Check sheet for the modelled part. Datum: model origin and axes. Units: mm. A direction names the side the tool comes from. Coordinates: 2 decimals unless noted, no trailing zeros. Loops run counter-clockwise (first coordinate to the right, second up) from the corner with the lowest first, then second, coordinate; pieces in that order, holes last.
Autodesk Inventor part; units mm, degrees
ref_plane "YZ Plane" through (0, 0, 0) normal (1, 0, 0) x (0, 1, 0)
ref_plane "XZ Plane" through (0, 0, 0) normal (0, 1, 0) x (-1, 0, 0)
ref_plane "XY Plane" through (0, 0, 0) normal (0, 0, 1) x (1, 0, 0)
sketch "Sketch1" plane through (0, 0, 0) normal (0, 0, 1) x (1, 0, 0)
  circle A0 centre (0, 0) radius 4
  line L0 (-0.0635, 3.5) -> (1.9365, 3.5)
  line L1 (-0.0635, 3.5) -> (2, 3.5) construction
  line L2 (1.9365, 3.5) -> (-1.9365, 3.5)
  line L3 (0, -3.5) -> (1.9365, -3.5)
  line L4 (1.9365, -3.5) -> (-1.9365, -3.5)
  dimension "d0" = 8
  dimension "d1" = 2
  dimension "d2" = 0
extrude "Extrusion1" add sketch "Sketch1" along normal blind 3 contours A0 L3 L4 L2 L0
sketch "Sketch2" plane through (0, 0, 3) normal (0, 0, 1) x (1, 0, 0)
  circle A0 centre (0, 0) radius 2.5
  dimension "d5" = 5
extrude "Extrusion2" add sketch "Sketch2" along normal blind 53
sketch "Sketch3" plane through (0, 0, 56) normal (0, 0, 1) x (1, 0, 0)
  arc A0 (-1.9365, 3.5) -> (-1.9365, -3.5) centre (0, 0) ccw
  circle A1 centre (0, 0) radius 2
  dimension "d8" = 4
extrude "Extrusion3" cut sketch "Sketch3" against normal blind 8
properties part number "Rotation Pin"
(1) Section check C-C, the plane z = 38. Enter the section's corners in (x, y).
(2) Scan lines: line 1 along Y through (x, z) = (0, 52.5); line 2 along Z through (x, y) = (2.75, 2); line 3 along Y through (x, z) = (0, 5.5). Record each from-to range of solid material in increasing order.
(3) Set-up check for faces 4 (the face through (-0.54, 2.44, 29.13)), 5 (the face through (0, 0, 0)): record each of +Z, -Z, +X, -X, +Y, -Y from which the full face is reachable in a straight line by a thin tool's end or side.
(4) Gauge pin test, flat ends, axial feed: P1, Ø1, axis at x = 2.5, z = 17.5, coming from the -Y side; P2, Ø4, axis at y = -2, z = 41, coming from the +X side; P3, Ø3, axis at x = 0, z = 32.5, coming from the -Y side; P4, Ø4, axis at x = 2, y = -1, coming from the -Z side. Record the tip position at first contact, or that the pin passes through.
(5) Section check B-B, the plane x = 0. Enter the section's corners in (y, z).
(6) Section check D-D, the plane x = -3.5. Enter the section's corners in (y, z), plus the area to 3 significant figures.
(7) Section check A-A, the plane y = 0. Enter the section's corners in (x, z), plus the area to 3 significant figures.
(8) Draft check along Y on faces 1 (the face through (-1, 2, 56)), 2 (the face through (0, -3.5, 1)), 3 (the face through (0, 0, 48)). Enter one of: pulls with the +Y half, pulls with the -Y half, needs draft (parallel to the pull), parting line crosses it, or undercut.
Determined:
1. outline: circle Ø5 at (0, 0)
2. line 1: y = -2.5 to -2, 2 to 2.5
2. line 2: z = 0 to 3
2. line 3: y = -2.5 to 2.5
3. face 4: +Z
3. face 5: -Z, +X, -X, +Y, -Y
4. P1: stops at y = -1.5
4. P2: stops at x = 2.5
4. P3: stops at y = -2.5
4. P4: stops at z = 0
5. outline: (-3.5, 0) - (3.5, 0) - (3.5, 3) - (2.5, 3) - (2.5, 56) - (2, 56) - (2, 48) - (-2, 48) - (-2, 56) - (-2.5, 56) - (-2.5, 3) - (-3.5, 3) - close
6. outline: (-1.94, 0) - (1.94, 0) - (1.94, 3) - (-1.94, 3) - close
6. area: 11.6 mm2
7. outline: (-4, 0) - (4, 0) - (4, 3) - (2.5, 3) - (2.5, 56) - (2, 56) - (2, 48) - (-2, 48) - (-2, 56) - (-2.5, 56) - (-2.5, 3) - (-4, 3) - close
7. area: 257 mm2
8. face 1: needs draft
8. face 2: pulls with the -Y half
8. face 3: undercut
